Part model, mm, in its own coordinate system. Give positions to 0.01 mm unless a question says otherwise; leave off trailing zeros. Order: outer loops, then holes, each group sorted by start corner. A loop starts at its lowest first (then second) coordinate and runs counter-clockwise, first axis right, second up. Notation, with made-up numbers: M 9.5,84 L 14.5,84 A15 cw 14.5,89 Z; hole C -40,17.5 d8. An arc over 180 degrees is marked long. Return JSON: item names as keys, results as strings.
from build123d import *

# Parameters (mm, degrees)
F0_W     = 60
F0_H     = 40
F1_DEPTH = 2
F2_R     = 3.343447
F2_R_2   = 4.664946
F2_R_3   = 5.011125
F3_DEPTH = 2
F4_R     = 5


with BuildPart() as f1:
    # F0 (on Top) → F1 (new body)
    with BuildSketch(Plane.XY):
        with Locations((2.640124, -1.107821)):
            Rectangle(F0_W, F0_H)
    extrude(amount=F1_DEPTH)

    # F2 (on face) → F3 (cut)
    with BuildSketch(Plane.XY.offset(2)):
        with Locations((-18.054973, 10.971558)):
            Circle(F2_R)
        with Locations((-18.267456, -9.115866)):
            Circle(F2_R_2)
        with Locations((10.761856, 7.836044)):
            Circle(F2_R_3)
    extrude(amount=-F3_DEPTH, mode=Mode.SUBTRACT)

    # F4
    f4_edges = [f1.edges().sort_by_distance(p)[0] for p in [
        (-27.359876, -21.107821, 1),
    ]]
    fillet(f4_edges, radius=F4_R)


solid = f1.part
Q1. Band-saw the part on B-B (y = -13). Give the cut face in (x, z).
Established:
{"outline": "M -27.36,0 L -20.85,0 L -20.85,2 L -27.36,2 Z; M -15.68,0 L 32.64,0 L 32.64,2 L -15.68,2 Z"}
Q2. Two-plate mould, pull along X, no slides. Class faces 1 (the cylindrical face through (-21.395, 11.119, 1.014)), 2 (the cylindrical face through (-22.928, -8.911, 1.014)), 3 (the flat face through (-27.36, 1, 1)), 4 (the flat face through (2, -1, 0)): +X half, -X half, draft (parallel to the pull), parting line (faces both ways), or undercut.
Established:
{"face 1": "undercut", "face 2": "undercut", "face 3": "-X half", "face 4": "draft"}
Q3. Band-saw the part on C-C (x = -17.5). Give the cut face in (y, z).
Established:
{"outline": "M -21.11,0 L -13.72,0 L -13.72,2 L -21.11,2 Z; M -4.51,0 L 7.67,0 L 7.67,2 L -4.51,2 Z; M 14.27,0 L 18.89,0 L 18.89,2 L 14.27,2 Z"}
Q4. Probe line 1 along Y through (x, z) = (-16, 0.45); line 2 along X through (y, z) = (3.5, 1.15); line 3 along Y through (x, z) = (-19, 0.35). List the from-to ranges inside material, lowest first.
Established:
{"line 1": "y = -21.11 to -13.19, -5.04 to 8.33, 13.61 to 18.89", "line 2": "x = -27.36 to 8.25, 13.27 to 32.64", "line 3": "y = -21.11 to -13.72, -4.51 to 7.76, 14.18 to 18.89"}
Q5. Band-saw the part on D-D (y = 9). Give the cut face in (x, z), then the cut area to 3 significant figures.
Established:
{"outline": "M -27.36,0 L -20.76,0 L -20.76,2 L -27.36,2 Z; M -15.35,0 L 5.89,0 L 5.89,2 L -15.35,2 Z; M 15.64,0 L 32.64,0 L 32.64,2 L 15.64,2 Z", "area": "89.7 mm²"}
Q6. Pin check, flat tip, straight feed: pin 1 (8 mm diameter, centred on x = 10.76, y = 7.84, fed in from -Z). Stop position of the tip, or through.
Established:
{"pin 1": "passes through"}
Q7. Band-saw the part on A-A (x = 11.5). Give the cut face in (y, z), then the cut area to 3 significant figures.
Established:
{"outline": "M -21.11,0 L 2.88,0 L 2.88,2 L -21.11,2 Z; M 12.79,0 L 18.89,0 L 18.89,2 L 12.79,2 Z", "area": "60.2 mm²"}
